Check sheet for the modelled part. Datum: model origin and axes. Units: mm. Face numbers are marked on the shaded views. A direction names the side the tool comes from. Coordinates: 2 decimals unless noted, no trailing zeros. Loops run counter-clockwise (first coordinate to the right, second up) from the corner with the lowest first, then second, coordinate; pieces in that order, holes last.
```python
from build123d import *

# Parameters (mm, degrees)
F1_DEPTH = 1.6
F3_DEPTH = 8
F4_R     = 0.6
F5_DEPTH = 8
F4_W     = 2.6
F4_H     = 2.6
F6_DEPTH = 6.2


with BuildPart() as f1:
    # F0 (on Top) → F1 (new body, symmetric)
    with BuildSketch(Plane.XY):
        with BuildLine():
            Line((-5, 0), (-3, 0))
            ThreePointArc((-3, 0), (-2.12132, 2.12132), (0, 3))
            Line((0, 3), (0, 10.2))
            Line((0, 10.2), (-22.7, 10.2))
            Line((-22.7, 10.2), (-22.7, 0))
            Line((-22.7, 0), (-21.8, 0))
            ThreePointArc((-21.8, 0), (-13.4, 8.4), (-5, 0))
        make_face()
        with BuildLine():
            ThreePointArc((0, -3), (-2.12132, -2.12132), (-3, 0))
            Line((-3, 0), (-5, 0))
            ThreePointArc((-5, 0), (-13.4, -8.4), (-21.8, 0))
            Line((-21.8, 0), (-22.7, 0))
            Line((-22.7, 0), (-22.7, -10.2))
            Line((-22.7, -10.2), (0, -10.2))
            Line((0, -10.2), (0, -3))
        make_face()
        with BuildLine():
            Line((0, 10.2), (0, 3))
            ThreePointArc((0, 3), (2.12132, 2.12132), (3, 0))
            Line((3, 0), (5, 0))
            ThreePointArc((5, 0), (13.4, 8.4), (21.8, 0))
            Line((21.8, 0), (22.7, 0))
            Line((22.7, 0), (22.7, 10.2))
            Line((22.7, 10.2), (0, 10.2))
        make_face()
        with BuildLine():
            ThreePointArc((3, 0), (2.12132, -2.12132), (0, -3))
            Line((0, -3), (0, -10.2))
            Line((0, -10.2), (22.7, -10.2))
            Line((22.7, -10.2), (22.7, 0))
            Line((22.7, 0), (21.8, 0))
            ThreePointArc((21.8, 0), (13.4, -8.4), (5, 0))
            Line((5, 0), (3, 0))
        make_face()
    extrude(amount=F1_DEPTH, both=True)

    # F2 (on face) → F3 (join)
    with BuildSketch(Plane.XY.offset(1.6)):
        Polygon((-22.7, 10.2), (0, 10.2), (0, 13.4), (-25.9, 13.4), (-25.9, -13.4), (0, -13.4), (0, -10.2), (-22.7, -10.2), align=None)
        Polygon((0, 10.2), (22.7, 10.2), (22.7, -10.2), (0, -10.2), (0, -13.4), (25.9, -13.4), (25.9, 13.4), (0, 13.4), align=None)
    extrude(amount=-F3_DEPTH)

    # F4 (on face) → F5 (join)
    with BuildSketch(Plane(origin=(0, 0, -1.6), x_dir=(1, 0, 0), z_dir=(0, 0, -1))):
        with Locations((-21.4, 8.9)):
            Circle(F4_R)
        with Locations((-21.4, -8.9)):
            Circle(F4_R)
        with Locations((21.4, -8.9)):
            Circle(F4_R)
        with Locations((21.4, 8.9)):
            Circle(F4_R)
    extrude(amount=F5_DEPTH)

    # F4 (on face) → F6 (join)
    with BuildSketch(Plane(origin=(0, 0, -1.6), x_dir=(1, 0, 0), z_dir=(0, 0, -1))):
        with Locations((-21.4, 8.9)):
            Rectangle(F4_W, F4_H)
        with Locations((-21.4, 8.9)):
            Circle(F4_R, mode=Mode.SUBTRACT)
        with Locations((-21.4, -8.9)):
            Rectangle(F4_W, F4_H)
        with Locations((-21.4, -8.9)):
            Circle(F4_R, mode=Mode.SUBTRACT)
        with Locations((21.4, 8.9)):
            Rectangle(F4_W, F4_H)
        with Locations((21.4, 8.9)):
            Circle(F4_R, mode=Mode.SUBTRACT)
        with Locations((21.4, -8.9)):
            Rectangle(F4_W, F4_H)
        with Locations((21.4, -8.9)):
            Circle(F4_R, mode=Mode.SUBTRACT)
    extrude(amount=F6_DEPTH)


solid = f1.part
```
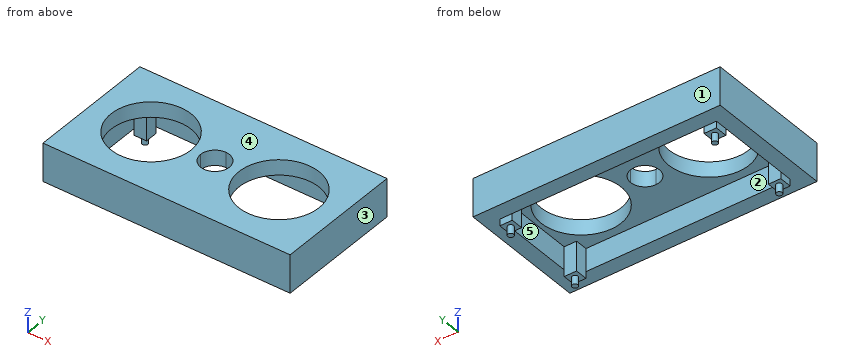
1) Section check A-A on z = -7.25. Enter the section's corners in (x, y).
Answer sheet:
outline: (-22.7, -10.2) - (-20.1, -10.2) - (-20.1, -7.6) - (-22.7, -7.6) - close; (-22.7, 7.6) - (-20.1, 7.6) - (-20.1, 10.2) - (-22.7, 10.2) - close; (20.1, -10.2) - (22.7, -10.2) - (22.7, -7.6) - (20.1, -7.6) - close; (20.1, 7.6) - (22.7, 7.6) - (22.7, 10.2) - (20.1, 10.2) - close
2) Scan lines: line 1 (X direction, y = -10, z = -2.75); line 2 (Y direction, x = 13.4, z = -0.85); line 3 (X direction, y = 4.5, z = -3). Record each from-to range of solid material in increasing order.
Answer sheet:
line 1: x = -25.9 to -20.1, 20.1 to 25.9
line 2: y = -13.4 to -8.4, 8.4 to 13.4
line 3: x = -25.9 to -22.7, 22.7 to 25.9
3) Section check C-C on y = -6.5. Enter the section's corners in (x, z).
Answer sheet:
outline: (-25.9, -6.4) - (-22.7, -6.4) - (-22.7, -1.6) - (-18.72, -1.6) - (-18.72, 1.6) - (-25.9, 1.6) - close; (-8.08, -1.6) - (8.08, -1.6) - (8.08, 1.6) - (-8.08, 1.6) - close; (18.72, -1.6) - (22.7, -1.6) - (22.7, -6.4) - (25.9, -6.4) - (25.9, 1.6) - (18.72, 1.6) - close
4) Depth check by flat-ended pin: pin 1 (3 mm diameter, centred on y = 9, z = -8, fed in from -X); pin 2 (1.1 mm diameter, centred on x = 22, z = -7, fed in from +Y); pin 3 (2 mm diameter, centred on x = 9, y = 7.5, fed in from -Z); pin 4 (1 mm diameter, centred on x = -15, y = 7.5, fed in from -Z). Enter the tip coordinate at first touch or a pass-through.
Answer sheet:
pin 1: stops at x = -22.7
pin 2: stops at y = 10.2
pin 3: stops at z = -1.6
pin 4: passes through
5) Section check D-D on z = 0.75. Enter the section's corners in (x, y), plus the area to 3 significant figures.
Answer sheet:
outline: (-25.9, -13.4) - (25.9, -13.4) - (25.9, 13.4) - (-25.9, 13.4) - close; hole circle Ø16.8 at (-13.4, 0); hole (-3, 0) arc R3 ccw to (0, -3) arc R3 ccw to (3, 0) arc R3 ccw to (0, 3) arc R3 ccw to start; hole circle Ø16.8 at (13.4, 0)
area: 917 mm2
6) Set-up check for the marked faces 1 and 2: record each of +Z, -Z, +X, -X, +Y, -Y from which the full face is reachable in a straight line by a thin tool's end or side.
Answer sheet:
face 1: +Z, -Z, +X, -X, +Y
face 2: -Z
7) Section check B-B on x = -13.4. Enter the section's corners in (y, z), plus the area to 3 significant figures.
Answer sheet:
outline: (-13.4, -6.4) - (-10.2, -6.4) - (-10.2, -1.6) - (-8.4, -1.6) - (-8.4, 1.6) - (-13.4, 1.6) - close; (8.4, -1.6) - (10.2, -1.6) - (10.2, -6.4) - (13.4, -6.4) - (13.4, 1.6) - (8.4, 1.6) - close
area: 62.7 mm2
8) Mould release check, pull along X, two halves, no side actions. Record for the marked faces 3, 4 and 5: +X half, -X half, draft (parallel to the pull), parting line (faces both ways), or undercut.
Answer sheet:
face 3: +X half
face 4: draft
face 5: undercut
